from build123d import *

# Parameters (mm, degrees)
SKETCH1_W           = 40
SKETCH1_H           = 50
BOSS_EXTRUDE1_DEPTH = 10
SKETCH2_W           = 40
SKETCH2_H           = 10
BOSS_EXTRUDE2_DEPTH = 20
FILLET1_R           = 10
SKETCH3_R           = 20
SKETCH3_R_2         = 15
BOSS_EXTRUDE3_DEPTH = 20
SKETCH4_R           = 5
CUT_EXTRUDE1_DEPTH  = 79.74007874


with BuildPart() as part:
    # Sketch1 → Boss-Extrude1 (new body)
    with BuildSketch(Plane.XY):
        Rectangle(SKETCH1_W, SKETCH1_H)
    extrude(amount=BOSS_EXTRUDE1_DEPTH)

    # Sketch2 → Boss-Extrude2 (add, symmetric)
    with BuildSketch(Plane(origin=(0, 0, 0), x_dir=(0, 0, -1), z_dir=(1, 0, 0))):
        with Locations((10, 30)):
            Rectangle(SKETCH2_W, SKETCH2_H)
        with Locations((10, -30)):
            Rectangle(SKETCH2_W, SKETCH2_H)
    extrude(amount=BOSS_EXTRUDE2_DEPTH, both=True)

    # Fillet1
    fillet1_edges = [part.edges().sort_by_distance(p)[0] for p in [
        (0, 35, 10),
        (-20, 30, -30),
        (20, 30, -30),
        (0, -35, 10),
        (-20, -30, -30),
        (20, -30, -30),
    ]]
    fillet(fillet1_edges, radius=FILLET1_R)

    # Sketch3 → Boss-Extrude3 (add)
    with BuildSketch(Plane.XY.offset(10)):
        Circle(SKETCH3_R)
        Circle(SKETCH3_R_2, mode=Mode.SUBTRACT)
    extrude(amount=BOSS_EXTRUDE3_DEPTH)

    # Sketch4 → Cut-Extrude1 (cut, through all)
    with BuildSketch(Plane.XZ.offset(35)):
        with Locations(Location((0, -20, 0), (0, 0, 270))):
            Circle(SKETCH4_R)
    extrude(amount=-CUT_EXTRUDE1_DEPTH, mode=Mode.SUBTRACT)


solid = part.part
Can you work these out from the model? Positions are in its coordinate system, mm. A direction names the side the tool comes from. Give positions to 0.01 mm unless a question says otherwise; leave off trailing zeros. Order: outer loops, then holes, each group sorted by start corner. A loop starts at its lowest first (then second) coordinate and runs counter-clockwise, first axis right, second up. Notation, with made-up numbers: M 9.5,49.5 L 26.5,49.5 A16 cw 26.5,73.5 Z; hole C 6,-27 d4. An arc over 180 degrees is marked long. Use a Markdown table: item, result. Add a question column.
Item 1: Will these pins go through, and if not, where does the flat tip stop? pin 1 (12 mm diameter, centred on x = -1, y = -13.5, fed in from -Z); pin 2 (3 mm diameter, centred on y = -8, z = 19.5, fed in from -X); pin 3 (6 mm diameter, centred on y = -16, z = 22, fed in from +X); pin 4 (1 mm diameter, centred on y = -23.5, z = -9, fed in from -X).
Item 2: Suppose I cut it at D-D (z = 12). List the corners of the cut face in (x, y) for me, then the cut area to 3 significant figures.
Item 3: We'd pull the mould along Z, two halves only. Please class faces 4 (the cylindrical face through (17.15, 30.07, -26.99)), 5 (the cylindrical face through (0, -30, -15)), 6 (the flat face through (0, 0, 10)): +Z half, -Z half, draft (parallel to the pull), parting line (faces both ways), or undercut.
Item 4: If I drill on L1, parallel to X at y = 30.75, z = -20; L2, parallel to Y at x = -7, z = -15; L3, parallel to Y at x = 0, z = 14.75, over which ranges is the centre line in solid material (lowest first)? Write a range as [from, to].
Item 5: Suppose I cut it at C-C (y = 26.5). List the corners of the cut face in (x, z) for me, then the cut area to 3 significant figures.
Item 6: Suppose I cut it at B-B (x = 0). List the corners of the cut face in (y, z) for me.
Item 7: For faces 1 (the flat face through (0.3, -25, -14.8)), 2 (the flat face through (0, -21, 10)), 3 (the cylindrical face through (-4.336, -19.524, 19.86)), which set-ups out of +Z, -Z, +X, -X, +Y, -Y let a thin tool reach every point of the face, with its end or its side?
Item 8: Suppose I cut it at A-A (z = -24). List the corners of the cut face in (x, y) for me, then the cut area to 3 significant figures.
Answer sheet:
| question | item | result |
|---|---|---|
| 1 | pin 1 | stops at z = 0 |
| 1 | pin 2 | stops at x = -18.91 |
| 1 | pin 3 | stops at x = 15.2 |
| 1 | pin 4 | passes through |
| 2 | outline | C 0,0 d40; hole C 0,0 d30 |
| 2 | area | 550 mm² |
| 3 | face 4 | -Z half |
| 3 | face 5 | undercut |
| 3 | face 6 | +Z half |
| 4 | L1 | x = [-20, -5], [5, 20] |
| 4 | L2 | y = [-35, -25], [25, 35] |
| 4 | L3 | y = [-20, -15], [15, 20] |
| 5 | outline | M -20,-20 A10 ccw -10,-30 L 10,-30 A10 ccw 20,-20 L 20,9.89 L -20,9.89 Z; hole C 0,-20 d10 |
| 5 | area | 1,470 mm² |
| 6 | outline | M -35,-30 L -25,-30 L -25,-25 L -35,-25 Z; M -35,-15 L -25,-15 L -25,0 L 25,0 L 25,-15 L 35,-15 L 35,0 A10 ccw 25,10 L 20,10 L 20,30 L 15,30 L 15,10 L -15,10 L -15,30 L -20,30 L -20,10 L -25,10 A10 ccw -35,0 Z; M 25,-30 L 35,-30 L 35,-25 L 25,-25 Z |
| 7 | face 1 | -Z, +X, -X |
| 7 | face 2 | +Z, -Y |
| 7 | face 3 | +Z |
| 8 | outline | M -19.17,-35 L -3,-35 L -3,-25 L -19.17,-25 Z; M -19.17,25 L -3,25 L -3,35 L -19.17,35 Z; M 3,-35 L 19.17,-35 L 19.17,-25 L 3,-25 Z; M 3,25 L 19.17,25 L 19.17,35 L 3,35 Z |
| 8 | area | 647 mm² |
